from build123d import *

# Parameters (mm, degrees)
SKETCH1_W                   = 10.16
SKETCH1_H                   = 41.91
BOSS_EXTRUDE1_DEPTH         = 17.78
SKETCH2_W                   = 10.16
SKETCH2_H                   = 27.178
CUT_EXTRUDE1_DEPTH          = 11.43
F_24_0_152_DIAMETER_HOLE1_D = 3.8608
FILLET1_R                   = 7.62
FILLET2_R                   = 2.54


with BuildPart() as part:
    # Sketch1 → Boss-Extrude1 (new body)
    with BuildSketch(Plane.XY):
        with Locations((5.08, 20.955)):
            Rectangle(SKETCH1_W, SKETCH1_H)
    extrude(amount=BOSS_EXTRUDE1_DEPTH)

    # Sketch2 → Cut-Extrude1 (cut)
    with BuildSketch(Plane.XY.offset(17.78)):
        with Locations((5.08, 20.955)):
            Rectangle(SKETCH2_W, SKETCH2_H)
    extrude(amount=-CUT_EXTRUDE1_DEPTH, mode=Mode.SUBTRACT)

    # #24 (0.152) Diameter Hole1 (through all)
    with Locations(Plane.XY.offset(17.78)):
        with Locations((5.08, 3.683), (5.08, 38.227)):
            Hole(F_24_0_152_DIAMETER_HOLE1_D / 2)

    # Fillet1
    fillet1_edges = [part.edges().sort_by_distance(p)[0] for p in [
        (5.08, 7.366, 6.35),
        (5.08, 34.544, 6.35),
    ]]
    fillet(fillet1_edges, radius=FILLET1_R)

    # Fillet2
    fillet2_edges = [part.edges().sort_by_distance(p)[0] for p in [
        (0, 20.955, 6.35),
        (10.16, 20.955, 6.35),
        (0, 7.366, 15.875),
        (10.16, 7.366, 15.875),
        (10.16, 34.544, 15.875),
        (0, 34.544, 15.875),
        (10.16, 9.597846327, 8.581846327),
        (0, 9.597846327, 8.581846327),
        (0, 32.312153673, 8.581846327),
        (10.16, 32.312153673, 8.581846327),
        (0, 41.91, 8.89),
        (10.16, 41.91, 8.89),
        (10.16, 0, 8.89),
        (0, 0, 8.89),
    ]]
    fillet(fillet2_edges, radius=FILLET2_R)


solid = part.part
Model file for the job. Use its own axes, mm. A direction names the side the tool comes from. Coordinates: 2 decimals unless noted, no trailing zeros. Order: outer loops, then holes, each group sorted by start corner. A loop starts at its lowest first (then second) coordinate and runs counter-clockwise, first axis right, second up. Notation, with made-up numbers: (19, -39) -> (40, -39) arc R29 ccw to (40, -8) -> close; hole circle Ø1 at (65.5, -10). An arc over 180 degrees is marked (long way). Return JSON: item names as keys, results as strings. Group by question number.
Item 1: Saw through at A-A on x = 5.08. Write the cut outline in (y, z).
Item 2: Wall check: line 1 along Y through (x, z) = (5.08, 5.75); line 2 along Y through (x, z) = (5.25, 6.25); line 3 along Y through (x, z) = (5.5, 15). Give the ranges that are in metal, low to high. Write a range as [from, to].
Item 3: Saw through at C-C on y = 3. Write the cut outline in (x, z), then the cut area to 3 significant figures.
Item 4: Tool access for faces 5 (the cylindrical face through (5.12, 32.37, 8.64)), 6 (the cylindrical face through (0.724, 21.039, 5.586)), 7 (the cylindrical face through (0.724, 41.146, 9.014)), 8 (the flat face through (5, 41.91, 9)), 9 (the cylindrical face through (9.4, 6.64, 15.85)): list every direction of +Z, -Z, +X, -X, +Y, -Y with a clear straight run to the whole face (end or side of a thin tool).
Item 5: Pull direction Y, two halves, no side cores. Call faces 1 (the cylindrical face through (9.396, 41.186, 9.014)), 2 (the flat face through (0, 21, 3)), 3 (the cylindrical face through (3.3, 2.94, 8.77)), 4 (the flat face through (5, 34.544, 16)): pulls with the +Y half, pulls with the -Y half, needs draft (parallel to the pull), parting line crosses it, or undercut.
Item 6: Flat gauge pins, fed straight in: P1, Ø3, axis at x = 8, y = 26.5, coming from the +Z side; P2, Ø3, axis at x = 6.5, y = 13, coming from the +Z side; P3, Ø4, axis at y = 23.5, z = 7, coming from the +X side. Where does each tip first touch, or does it go through?
Item 7: Saw through at B-B on z = 12. State how many separate pieces and enclosed holes the cut face has, then the cut area to 3 significant figures.
Values found:
{
 "1": {"outline": "(0, 0) -> (1.75, 0) -> (1.75, 17.78) -> (0, 17.78) -> close; (5.61, 0) -> (36.3, 0) -> (36.3, 17.78) -> (34.54, 17.78) -> (34.54, 13.97) arc R7.62 cw to (26.92, 6.35) -> (14.99, 6.35) arc R7.62 cw to (7.37, 13.97) -> (7.37, 17.78) -> (5.61, 17.78) -> close; (40.16, 0) -> (41.91, 0) -> (41.91, 17.78) -> (40.16, 17.78) -> close"},
 "2": {"line 1": "y = [0, 1.75], [5.61, 36.3], [40.16, 41.91]", "line 2": "y = [0, 1.76], [5.61, 36.3], [40.15, 41.91]", "line 3": "y = [0, 1.8], [5.57, 7.37], [34.54, 36.34], [40.11, 41.91]"},
 "3": {"outline": "(0, 0) -> (3.27, 0) -> (3.27, 17.78) -> (0, 17.78) -> close; (6.89, 0) -> (10.16, 0) -> (10.16, 17.78) -> (6.89, 17.78) -> close", "area": "116 mm2"},
 "4": {"face 5": "+Z, +X, -X", "face 6": "+Z, -X", "face 7": "+Z, -Z, -X, +Y", "face 8": "+Z, -Z, +X, -X, +Y", "face 9": "+Z, +X"},
 "5": {"face 1": "pulls with the +Y half", "face 2": "needs draft", "face 3": "undercut", "face 4": "undercut"},
 "6": {"P1": "stops at z = 6.42", "P2": "stops at z = 7.19", "P3": "stops at x = 9.86"},
 "7": {"separate pieces": "2", "enclosed holes": "2", "area": "120 mm2"}
}
